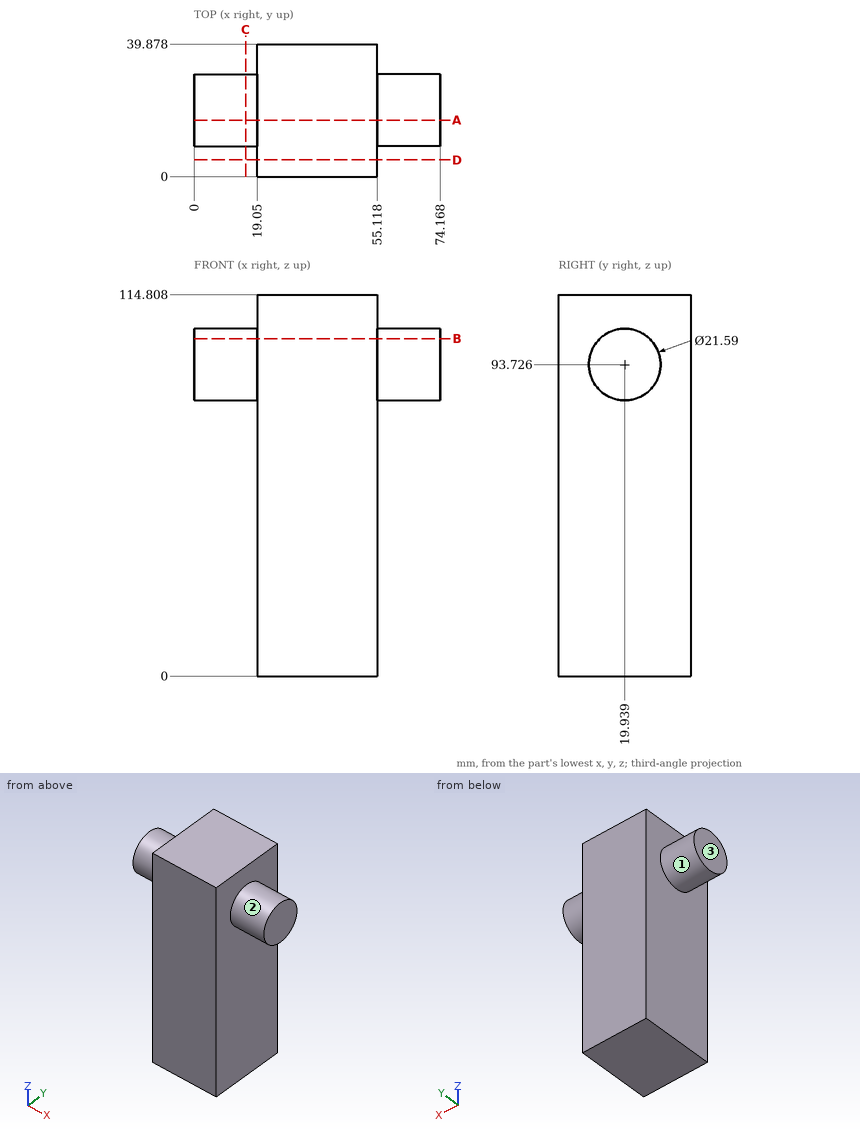
Answer from the drawing. Dimensions are ordinates in mm from the lowest x, y and z of the part. A direction names the side the tool comes from. Give positions to 0.01 mm unless a question says otherwise; leave off trailing zeros. Loops run counter-clockwise (first coordinate to the right, second up) from the corner with the lowest first, then second, coordinate; pieces in that order, holes last. Notation, with made-up numbers: (-6.5, 66) - (22.5, 66) arc R17 cw to (22.5, 90) - close; hole circle Ø11 at (7.25, 6). An arc over 180 degrees is marked (long way). Write each question's results on one line, items separated by ' | '.
1. Find section C-C, the plane x = 15.5. Write down the section's boundary in (y, z) (3 decimals).
Resolved:
outline: circle Ø21.59 at (19.939, 93.726)
2. Find section A-A, the plane y = 17. Write down the section's boundary in (x, z).
Resolved:
outline: (0, 83.34) - (19.05, 83.34) - (19.05, 0) - (55.12, 0) - (55.12, 83.34) - (74.17, 83.34) - (74.17, 104.11) - (55.12, 104.11) - (55.12, 114.81) - (19.05, 114.81) - (19.05, 104.11) - (0, 104.11) - close
3. Flat-ended cylindrical pins translate along their axes: P1, Ø2, axis at y = 33, z = 48, coming from the -X side; P2, Ø8, axis at y = 27.5, z = 32, coming from the +X side; P3, Ø6, axis at x = 14.5, y = 13.5, coming from the -Z side. Find the tip coordinate at first contact, or state that the pin passes through.
Resolved:
P1: stops at x = 19.05 | P2: stops at x = 55.12 | P3: stops at z = 83.49
4. Consider probe 1 along X at (y, z) = (15, 33); probe 2 along Z at (x, y) = (70.5, 12); probe 3 along Y at (x, z) = (66, 103). Determine where each line is inside the solid, lowest interval first. Write a range as from..to.
Resolved:
probe 1: x = 19.05..55.12 | probe 2: z = 86.41..101.04 | probe 3: y = 14.41..25.46
5. Find section B-B, the plane z = 101.5. Write down the section's boundary in (x, y), then the cut area to 3 significant figures.
Resolved:
outline: (0, 12.45) - (19.05, 12.45) - (19.05, 0) - (55.12, 0) - (55.12, 12.45) - (74.17, 12.45) - (74.17, 27.43) - (55.12, 27.43) - (55.12, 39.88) - (19.05, 39.88) - (19.05, 27.43) - (0, 27.43) - close | area: 2,010 mm^2
6. Find section D-D, the plane y = 5. Write down the section's boundary in (x, z), then the cut area to 3 significant figures.
Resolved:
outline: (19.05, 0) - (55.12, 0) - (55.12, 114.81) - (19.05, 114.81) - close | area: 4,140 mm^2
7. Which of the six approach directions +Z, -Z, +X, -X, +Y, -Y give full straight-line access (tool end or side, diameter ignored) to the marked faces 1, 2 and 3?
Resolved:
face 1: -X | face 2: +X | face 3: +Z, -Z, -X, +Y, -Y
